from build123d import *

# Parameters (mm, degrees)
SKETCH1_W           = 38
SKETCH1_H           = 8.3
BOSS_EXTRUDE1_DEPTH = 3.05
SKETCH3_W           = 3
SKETCH3_H           = 1
CUT_EXTRUDE2_DEPTH  = 40.015285466
CUT_EXTRUDE1_DEPTH  = 40.015285466
FILLET1_R           = 0.5
SKETCH4_W           = 38
SKETCH4_H           = 3.05
BOSS_EXTRUDE2_DEPTH = 7


with BuildPart() as part:
    # Sketch1 → Boss-Extrude1 (new body)
    with BuildSketch(Plane(origin=(0, 0, 0), x_dir=(1, 0, 0), z_dir=(0, 1, 0))):
        with Locations((19, 4.15)):
            Rectangle(SKETCH1_W, SKETCH1_H)
    extrude(amount=BOSS_EXTRUDE1_DEPTH)

    # Sketch3 → Cut-Extrude2 (cut, through all)
    with BuildSketch(Plane(origin=(0, 3.05, 0), x_dir=(1, 0, 0), z_dir=(0, 1, 0))):
        Polygon((20.65, 4.1), (19, 4.1), (17.35, 4.1), (17.35, 0), (20.65, 0), align=None)
        with Locations((19, 5.8)):
            Rectangle(SKETCH3_W, SKETCH3_H)
    extrude(amount=-CUT_EXTRUDE2_DEPTH, mode=Mode.SUBTRACT)

    # Sketch2 → Cut-Extrude1 (cut, through all)
    with BuildSketch(Plane(origin=(0, 3.05, 0), x_dir=(1, 0, 0), z_dir=(0, 1, 0))):
        Polygon((4.425, 2), (6, 0), (11.35, 0), (12.925, 2), align=None)
        Polygon((33.575, 2), (25.075, 2), (26.65, 0), (32, 0), align=None)
    extrude(amount=-CUT_EXTRUDE1_DEPTH, mode=Mode.SUBTRACT)

    # Fillet1
    fillet1_edges = [part.edges().sort_by_distance(p)[0] for p in [
        (12.925, 1.525, -2),
        (11.35, 1.525, 0),
        (6, 1.525, 0),
        (4.425, 1.525, -2),
        (33.575, 1.525, -2),
        (32, 1.525, 0),
        (26.65, 1.525, 0),
        (25.075, 1.525, -2),
    ]]
    fillet(fillet1_edges, radius=FILLET1_R)

    # Sketch4 → Boss-Extrude2 (add)
    with BuildSketch(Plane(origin=(0, 0, -8.3), x_dir=(-1, 0, 0), z_dir=(0, 0, -1))):
        with Locations((-19, 1.525)):
            Rectangle(SKETCH4_W, SKETCH4_H)
    extrude(amount=BOSS_EXTRUDE2_DEPTH)


solid = part.part
Check sheet for the modelled part. Datum: model origin and axes. Units: mm. A direction names the side the tool comes from. Round coordinates to 2 decimals unless told otherwise and drop trailing zeros. Loops run counter-clockwise (first coordinate to the right, second up) from the corner with the lowest first, then second, coordinate; pieces in that order, holes last. Notation, with made-up numbers: (-26.75, 39.25) - (29.25, 39.25) arc R24 cw to (29.25, 64.25) - close; hole circle Ø1 at (16, -2). An arc over 180 degrees is marked (long way). Answer as CSV lines item,"result". Start each with the question number.
Item 1: Section check C-C (x = 28). Record the boundary of the cut face in (y, z), and give its area (3 significant figures).
Item 2: Release check for a two-part mould opening along X. For faces 4 (the flat face through (19, 2, -4.1)), 5 (the flat face through (19, 3.05, -8)), 6 (the flat face through (0, 2, -8)) record: +X half, -X half, draft (parallel to the pull), parting line (faces both ways), or undercut.
Item 3: Set-up check for faces 1 (the cylindrical face through (32.584, 1.504, -0.275)), 2 (the flat face through (35, 2, 0)), 3 (the flat face through (20.65, 2, -2)): record each of +Z, -Z, +X, -X, +Y, -Y from which the full face is reachable in a straight line by a thin tool's end or side.
Item 4: Scan lines: line 1 (X direction, y = 2.1, z = -1.5); line 2 (X direction, y = 2.55, z = -3); line 3 (Z direction, x = 19.5, y = 0.3). Record each from-to range of solid material in increasing order. Write a range as [from, to].
Item 5: Section check A-A (y = 2.3). Record the boundary of the cut face in (x, z).
Item 6: Section check B-B (x = 18.5). Record the boundary of the cut face in (y, z).
Report:
1,outline,"(0, -15.3) - (3.05, -15.3) - (3.05, -2) - (0, -2) - close"
1,area,"40.6 mm2"
2,face 4,"undercut"
2,face 5,"draft"
2,face 6,"-X half"
3,face 1,"+Y, -Y"
3,face 2,"+Z, +X, -X, +Y, -Y"
3,face 3,"+Z, +Y, -Y"
4,line 1,"x = [0, 4.96], [12.39, 17.35], [20.65, 25.61], [33.04, 38]"
4,line 2,"x = [0, 17.35], [20.65, 38]"
4,line 3,"z = [-15.3, -6.3], [-5.3, -4.1]"
5,outline,"(0, -15.3) - (38, -15.3) - (38, 0) - (33.03, 0) arc R0.5 ccw to (32.64, -0.81) - (32.94, -1.19) arc R0.5 cw to (32.54, -2) - (26.11, -2) arc R0.5 cw to (25.71, -1.19) - (26.01, -0.81) arc R0.5 ccw to (25.62, 0) - (20.65, 0) - (20.65, -4.1) - (17.35, -4.1) - (17.35, 0) - (12.38, 0) arc R0.5 ccw to (11.99, -0.81) - (12.29, -1.19) arc R0.5 cw to (11.89, -2) - (5.46, -2) arc R0.5 cw to (5.06, -1.19) - (5.36, -0.81) arc R0.5 ccw to (4.97, 0) - (0, 0) - close; hole (17.5, -6.3) - (20.5, -6.3) - (20.5, -5.3) - (17.5, -5.3) - close"
6,outline,"(0, -15.3) - (3.05, -15.3) - (3.05, -6.3) - (0, -6.3) - close; (0, -5.3) - (3.05, -5.3) - (3.05, -4.1) - (0, -4.1) - close"
